Answer from the drawing. Dimensions are ordinates in mm from the lowest x, y and z of the part. Coordinates: 2 decimals unless noted, no trailing zeros. Write each loop counter-clockwise with the first axis right and the second up, starting at its lowest first coordinate (ties: lowest second). Pieces come first, ordered by that corner, then holes. Notation, with made-up numbers: (73, 21) -> (89, 21) arc R31 ccw to (89, 48) -> close; hole circle Ø8 at (64, 88.25). An arc over 180 degrees is marked (long way). Use CSV: the item, a comma, the result in double quotes.
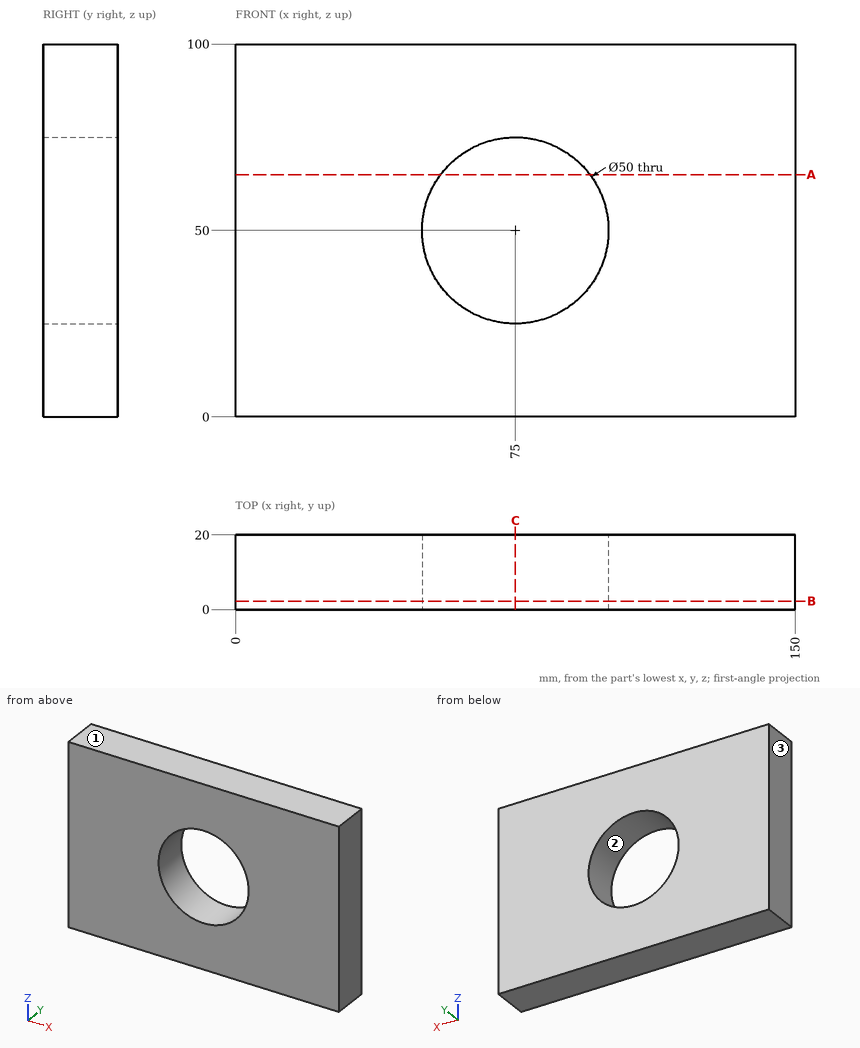
1. For a pull along Z with two mould halves and no side action, classify the marked faces 1, 2 and 3 as pulls with the +Z half, pulls with the -Z half, needs draft (parallel to the pull), parting line crosses it, or undercut.
Solutions:
face 1,"pulls with the +Z half"
face 2,"undercut"
face 3,"needs draft"
2. A cutting plane is placed at C-C (x = 75). Give the vertices of the cut face in (y, z).
Solutions:
outline,"(0, 0) -> (20, 0) -> (20, 25) -> (0, 25) -> close; (0, 75) -> (20, 75) -> (20, 100) -> (0, 100) -> close"
3. Find the intervals of material crossed by line 1 along Z through (x, y) = (75, 15.25); line 2 along X through (y, z) = (8.75, 47); line 3 along Z through (x, y) = (63, 9.5), in increasing order.
Solutions:
line 1,"z = 0 to 25, 75 to 100"
line 2,"x = 0 to 50.18, 99.82 to 150"
line 3,"z = 0 to 28.07, 71.93 to 100"
4. This flat-tipped pin is pushed along its axis until it touches: pin 1 Ø8 at (x, z) = (131.5, 81.5) entering from -Y. Where does it stop, or does it pass through?
Solutions:
pin 1,"stops at y = 0"
5. A cutting plane is placed at B-B (y = 2.25). Give the vertices of the cut face in (x, z).
Solutions:
outline,"(0, 0) -> (150, 0) -> (150, 100) -> (0, 100) -> close; hole circle Ø50 at (75, 50)"
6. A cutting plane is placed at A-A (z = 65). Give the vertices of the cut face in (x, y), and give its area (3 significant figures).
Solutions:
outline,"(0, 0) -> (55, 0) -> (55, 20) -> (0, 20) -> close; (95, 0) -> (150, 0) -> (150, 20) -> (95, 20) -> close"
area,"2,200 mm^2"
